Autodesk Inventor part; units mm, degrees
ref_plane "Work Plane1" through (15, 0, 0) normal (-1, 0, 0) x (0, 0, 1)
ref_plane "Work Plane2" through (15, 0, 0) normal (1, 0, 0) x (0, 0, -1)
ref_plane "Work Plane3" through (0, 40, 0) normal (0, 1, 0) x (-1, 0, 0)
sketch "Sketch3" plane through (0, 0, 0) normal (1, 0, 0) x (0, 1, 0)
  circle A0 centre (0, 0) radius 40
  circle A1 centre (0, 0) radius 5
  dimension "d2" = 80
  dimension "d3" = 10
extrude "Extrusion1" add sketch "Sketch3" along normal blind 30 contours A0 | A1
sketch "Sketch4" plane through (30, 0, 0) normal (1, 0, 0) x (0, 0, -1)
  circle A0 centre (0, 0) radius 5 construction
  circle A1 centre (0, 0) radius 36
  circle A2 centre (0, 0) radius 40
  dimension "d6" = 4
ref_plane "Work Plane1" through (15, 0, 0) normal (-1, 0, 0) x (0, 0, 1)
extrude "Extrusion2" cut sketch "Sketch4" against normal blind 10 contours A1
sketch "Sketch5" plane through (20, 0, 0) normal (1, 0, 0) x (0, 0, -1)
  circle A0 centre (0, 0) radius 4
  circle A1 centre (0, 0) radius 36 construction
  dimension "d12" = 8
extrude "Extrusion3" cut sketch "Sketch5" against normal up to next
sketch "Sketch6" plane through (20, 0, 0) normal (1, 0, 0) x (0, 0, -1)
  circle A0 centre (0, 0) radius 4
  circle A1 centre (0, 0) radius 36
  line L0 (-10, 10) -> (10, 10)
  line L1 (10, 10) -> (10, -10)
  line L2 (10, -10) -> (-10, -10)
  line L3 (-10, -10) -> (-10, 10)
  line L4 (-10, 10) -> (10, -10) construction
  line L5 (10, 10) -> (-10, -10) construction
  dimension "d13" = 20
extrude "Extrusion4" add sketch "Sketch6" along normal up to surface (10 mm away) contours A1
ref_plane "Work Plane2" through (15, 0, 0) normal (1, 0, 0) x (0, 0, -1)
sketch "Sketch7" plane through (30, 0, 0) normal (1, 0, 0) x (0, 0, -1)
  circle A0 centre (0, 0) radius 36
extrude "Extrusion5" cut sketch "Sketch7" against normal blind 5
sketch "Sketch8" plane through (0, 0, 0) normal (-1, 0, 0) x (0, 0, 1)
  circle A0 centre (0, 0) radius 36
  circle A1 centre (0, 0) radius 4
extrude "Extrusion6" cut sketch "Sketch8" against normal blind 15
sketch "Sketch9" plane through (15, 0, 0) normal (-1, 0, 0) x (0, 0, 1)
  circle A0 centre (0, 0) radius 4
  circle A1 centre (0, 0) radius 10
  dimension "d21" = 20
extrude "Extrusion7" add sketch "Sketch9" along normal blind 25
sketch "Sketch10" plane through (15, 0, 0) normal (-1, 0, 0) x (0, 0, 1)
  line L0 (0, 0) -> (28.2843, 28.2843)
  line L1 (0, 0) -> (-28.2843, 28.2843)
  circle A0 centre (0, 0) radius 40
  circle A1 centre (0, 0) radius 4 construction
  line L2 (0, 0) -> (0, 40) construction
  dimension "d24" = 90
ref_plane "Work Plane3" through (0, 40, 0) normal (0, 1, 0) x (-1, 0, 0)
properties part number "wheel" material "Aluminum 6061"
The listing builds one solid part. Answer for the finished solid, in the listing's coordinates (mm). A direction names the side the tool comes from. Round coordinates to 2 decimals unless told otherwise and drop trailing zeros. Loops run counter-clockwise (first coordinate to the right, second up) from the corner with the lowest first, then second, coordinate; pieces in that order, holes last. Notation, with made-up numbers: (27, -12.75) - (57, -12.75) arc R18 cw to (57, -7.75) - close; hole circle Ø3 at (-9, -6.5). An arc over 180 degrees is marked (long way). Return JSON: item names as keys, results as strings. Group by question number.
1. The part is cut by section C-C on x = -5.5. Determine the outline of the cut face in (y, z), then the cut area to 3 significant figures.
2. The mould has two halves that part along Z. Classify faces 1 (the cylindrical face through (27.535, 35.694, 4.686)), 2 (the flat face through (30, 15, 33)), 3 (the flat face through (25, -15, 1)), 4 (the cylindrical face through (14.79, -8.67, 39.05)): pulls with the +Z half, pulls with the -Z half, needs draft (parallel to the pull), parting line crosses it, or undercut.
3. The part is cut by section A-A on z = 0. Determine the outline of the cut face in (x, y).
4. The part is cut by section D-D on y = 21. Determine the outline of the cut face in (x, z).
5. Each of these flat-tipped pins is pushed along its axis until it touches: P1, Ø5, axis at x = 11, y = -21, coming from the +Z side; P2, Ø2.5, axis at x = 23, y = 1.5, coming from the -Z side; P3, Ø3, axis at y = 22, z = 26.5, coming from the +X side; P4, Ø6.5, axis at y = 0, z = 0, coming from the +X side. Where does it stop, or does it pass through?
6. Which of the six approach directions +Z, -Z, +X, -X, +Y, -Y give full straight-line access (tool end or side, diameter ignored) to faces 5 (the cylindrical face through (2.68, 9.76, -2.17)), 6 (the flat face through (-10, 0.1, 4.3)), 7 (the flat face through (20, 0.1, -4.3))?
7. Consider probe 1 along Z at (x, y) = (11.5, -8.5); probe 2 along Z at (x, y) = (5, -3); probe 3 along X at (y, z) = (11, 0). Determine where each line is inside the solid, lowest interval first.
Resolved:
{
 "1": {"outline": "circle Ø20 at (0, 0); hole circle Ø8 at (0, 0)", "area": "264 mm²"},
 "2": {"face 1": "undercut", "face 2": "needs draft", "face 3": "undercut", "face 4": "parting line crosses it"},
 "3": {"outline": "(-10, -10) - (15, -10) - (15, -36) - (0, -36) - (0, -40) - (30, -40) - (30, -36) - (25, -36) - (25, -10) - (20, -10) - (20, -4) - (-10, -4) - close; (-10, 4) - (20, 4) - (20, 10) - (25, 10) - (25, 36) - (30, 36) - (30, 40) - (0, 40) - (0, 36) - (15, 36) - (15, 10) - (-10, 10) - close"},
 "4": {"outline": "(0, -34.04) - (30, -34.04) - (30, -29.24) - (25, -29.24) - (25, 29.24) - (30, 29.24) - (30, 34.04) - (0, 34.04) - (0, 29.24) - (15, 29.24) - (15, -29.24) - (0, -29.24) - close"},
 "5": {"P1": "stops at z = 35.46", "P2": "stops at z = -40", "P3": "stops at x = 25", "P4": "passes through"},
 "6": {"face 5": "-X", "face 6": "+Z, -Z, -X, +Y, -Y", "face 7": "+X"},
 "7": {"probe 1": "z = -39.09 to -34.98, -5.27 to 5.27, 34.98 to 39.09", "probe 2": "z = -39.89 to -35.87, -9.54 to -2.65, 2.65 to 9.54, 35.87 to 39.89", "probe 3": "x = 15 to 25"}
}
